Print and shaded views of the part. All mm, measured from the part's lowest x, y and z. A direction names the side the tool comes from. Round coordinates to 2 decimals unless told otherwise and drop trailing zeros. Order: outer loops, then holes, each group sorted by start corner. A loop starts at its lowest first (then second) coordinate and runs counter-clockwise, first axis right, second up. Notation, with made-up numbers: (-30, 8.25) - (10, 8.25) arc R31 ccw to (10, 39.25) - close; hole circle Ø9 at (72.5, 4.25). An arc over 180 degrees is marked (long way). Return JSON: item names as keys, results as strings. Group by question number.
Item 1: Tool access for the marked faces 4, 5 and 6: list every direction of +Z, -Z, +X, -X, +Y, -Y with a clear straight run to the whole face (end or side of a thin tool).
Item 2: Drop flat-ended pins along their axis: pin 1 (5 mm diameter, centred on x = 25, y = 63.91, fed in from +Z); pin 2 (1 mm diameter, centred on y = 54, z = 2.5, fed in from +X). Give the stop position or say it passes through.
Item 3: Saw through at A-A on z = 3.75. List the corners of the cut face in (x, y) (1 decimal), and give its area (3 significant figures).
Item 4: Saw through at B-B on x = 25. List the corners of the cut face in (y, z) (1 decimal), and give its area (3 significant figures).
Item 5: Saw through at D-D on y = 13.5. List the corners of the cut face in (x, z), and give its area (3 significant figures).
Item 6: Two-plate mould, pull along Y, no slides. Class the marked faces 1, 2 and 3: released by +Y, released by -Y, zero draft, split by the parting line, or undercut.
Item 7: Saw through at C-C on x = 3. List the corners of the cut face in (y, z) (1 decimal).
Item 8: Probe probe 1 along X at (y, z) = (2.6, 3.75) (1 decimal); probe 2 along Y at (x, z) = (38, 4.5) (1 decimal); probe 3 along X at (y, z) = (60.5, 5.75). List the from-to ranges inside material, lowest first.
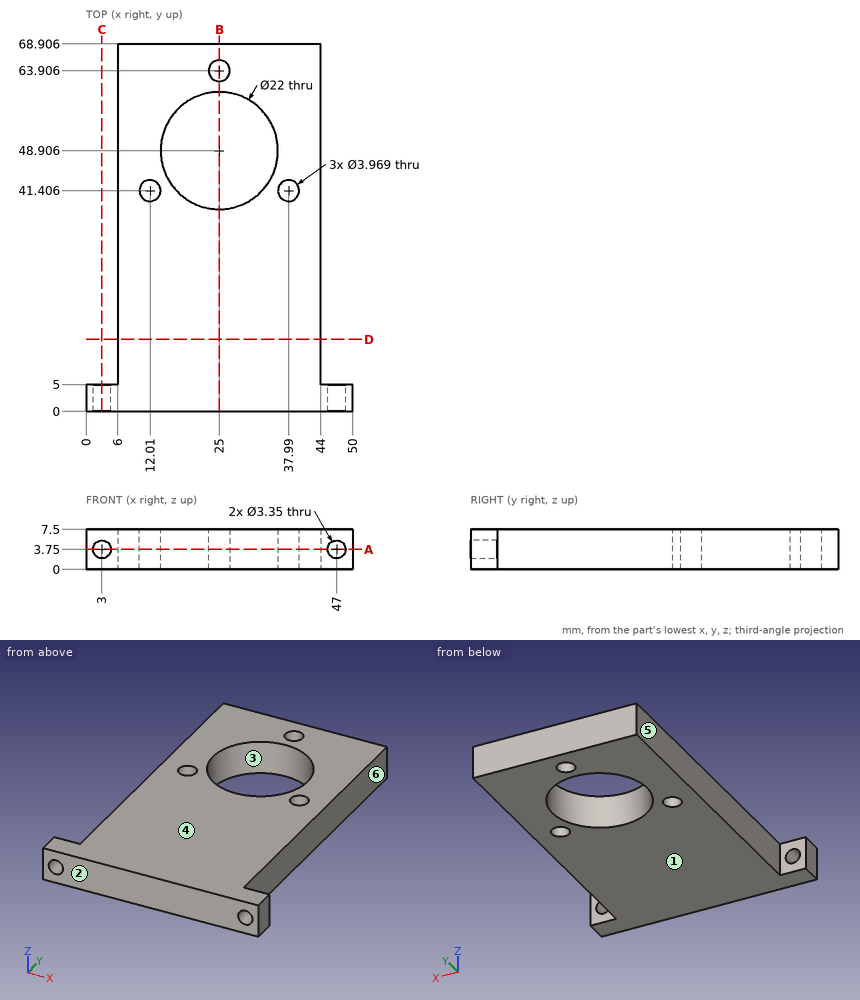
Filled in:
{
 "1": {"face 4": "+Z, +X, -X, +Y, -Y", "face 5": "+Z, -Z, -X, +Y", "face 6": "+Z, -Z, +X, +Y"},
 "2": {"pin 1": "stops at z = 7.5", "pin 2": "stops at x = 44"},
 "3": {"outline": "(0, 0) - (1.3, 0) - (1.3, 5) - (0, 5) - close; (4.7, 0) - (45.3, 0) - (45.3, 5) - (44, 5) - (44, 68.9) - (6, 68.9) - (6, 5) - (4.7, 5) - close; (48.7, 0) - (50, 0) - (50, 5) - (48.7, 5) - close; hole circle Ø4 at (12, 41.4); hole circle Ø22 at (25, 48.9); hole circle Ø4 at (25, 63.9); hole circle Ø4 at (38, 41.4)", "area": "2,230 mm^2"},
 "4": {"outline": "(0, 0) - (37.9, 0) - (37.9, 7.5) - (0, 7.5) - close; (59.9, 0) - (61.9, 0) - (61.9, 7.5) - (59.9, 7.5) - close; (65.9, 0) - (68.9, 0) - (68.9, 7.5) - (65.9, 7.5) - close", "area": "322 mm^2"},
 "5": {"outline": "(6, 0) - (44, 0) - (44, 7.5) - (6, 7.5) - close", "area": "285 mm^2"},
 "6": {"face 1": "zero draft", "face 2": "released by -Y", "face 3": "undercut"},
 "7": {"outline": "(0, 0) - (5, 0) - (5, 2.1) - (0, 2.1) - close; (0, 5.4) - (5, 5.4) - (5, 7.5) - (0, 7.5) - close"},
 "8": {"probe 1": "x = 0 to 1.3, 4.7 to 45.3, 48.7 to 50", "probe 2": "y = 0 to 39.4, 43.4 to 68.9", "probe 3": "x = 6 to 44"}
}
